Source: CAD feature listing. Evaluate the final solid. Frame: model axes, mm. A direction names the side the tool comes from. Coordinates: 2 decimals unless noted, no trailing zeros. Order: outer loops, then holes, each group sorted by start corner. A loop starts at its lowest first (then second) coordinate and runs counter-clockwise, first axis right, second up.
Autodesk Inventor part; units mm, degrees
ref_plane "YZ Plane" through (0, 0, 0) normal (1, 0, 0) x (0, 1, 0)
ref_plane "XZ Plane" through (0, 0, 0) normal (0, 1, 0) x (-1, 0, 0)
ref_plane "XY Plane" through (0, 0, 0) normal (0, 0, 1) x (1, 0, 0)
sketch "Sketch1" plane through (0, 0, 0) normal (0, 1, 0) x (-1, 0, 0)
  line L0 (0, 0) -> (0, -228.6)
  line L1 (0, -228.6) -> (-25.4, -228.6)
  line L2 (-25.4, -228.6) -> (-25.4, 10.5159)
  line L3 (-25.4, 10.5159) -> (24.2621, 60.178)
  line L4 (24.2621, 60.178) -> (42.5226, 42.5226)
  line L5 (42.5226, 42.5226) -> (0, 0)
  dimension "d0" = 228.6
  dimension "d1" = 25.4
  dimension "d2" = 135
  dimension "d3" = 25.4
extrude "Extrusion1" add sketch "Sketch1" along normal blind 25.4
sketch "Sketch2" plane through (0, 25.4, 0) normal (0, 1, 0) x (1, 0, 0)
  line L0 (25.4, 228.6) -> (0, 228.6)
  line L1 (9.525, 228.6) -> (0, 182.5245)
  line L2 (0, 228.6) -> (0, 0)
  dimension "d6" = 11.68
  dimension "d7" = 9.525
extrude "Extrusion2" cut sketch "Sketch2" against normal through all
shell "Shell1" thickness 3.175 removed faces 3 at (3.175, 16.9333, -197.883) at (14.8167, 8.4667, -228.6) at (-30.3489, 8.4667, 54.2929)
sketch "Sketch3" plane through (0, 25.4, 0) normal (0, 1, 0) x (1, 0, 0)
  circle A0 centre (-24.4095, -42.3701) radius 3.175
  line L0 (-42.5226, -42.5226) -> (-24.2621, -60.178)
  line L1 (0, 0) -> (-42.5226, -42.5226)
  line L2 (0, 0) -> (25.4, 0)
  line L3 (25.4, -10.5159) -> (25.4, 228.6)
  circle A1 centre (12.7, 12.7) radius 2.54
  line L4 (0, 182.5245) -> (0, 0)
  dimension "d11" = 6.35
  dimension "d12" = 12.7
  dimension "d13" = 12.7
  dimension "d14" = 5.08
  dimension "d15" = 12.7
  dimension "d16" = 12.7
extrude "Extrusion3" cut sketch "Sketch3" against normal through all
properties material "Aluminum 6061"
1. Section query C-C on x = 12.7. Return loops of the section in (y, z) (3 decimals).
Findings:
outline: (0, -228.6) - (3.175, -228.6) - (3.175, -15.24) - (0, -15.24) - close; (0, -10.16) - (3.175, -10.16) - (3.175, 18.726) - (22.225, 18.726) - (22.225, -10.16) - (25.4, -10.16) - (25.4, 23.216) - (0, 23.216) - close; (22.225, -228.6) - (25.4, -228.6) - (25.4, -15.24) - (22.225, -15.24) - close
2. Section query B-B on y = 8. Return loops of the section in (x, z) (1 decimal).
Findings:
outline: (-42.5, 42.5) - (0, 0) - (0, -182.5) - (3.2, -197.9) - (3.2, 1.3) - (-40.2, 44.7) - close; (-26.5, 58) - (22.2, 9.2) - (22.2, -228.6) - (25.4, -228.6) - (25.4, 10.5) - (-24.3, 60.2) - close
3. Access query for faces 1 (the face through (12.37, 23.83, -15.22)), 2 (the face through (22.225, 13, -111)), 3 (the face through (0, 13, -90)), 4 (the face through (7, 3.175, -85)). Directions: +Z, -Z, +X, -X, +Y, -Y. A direction counts if a zero-diameter tool reaches every point of the face in a straight line with its end or side. Return the directions, or none.
Findings:
face 1: +Y, -Y
face 2: -Z
face 3: -Z, -X, +Y, -Y
face 4: none
4. Pin query (flat end, axial travel): P1, Ø2, axis at y = 19.5, z = -152, coming from the -X side; P2, Ø6, axis at y = 21, z = 18.5, coming from the -X side; P3, Ø10, axis at x = 13, y = 4, coming from the +Z side. Return the tip coordinate at first contact, or that it passes through.
Findings:
P1: stops at x = 0
P2: stops at x = -21.5
P3: stops at z = 27.92
5. Section query D-D on x = -31. Return loops of the section in (y, z) (3 decimals), plus the area to 3 significant figures.
Findings:
outline: (0, 31) - (25.4, 31) - (25.4, 53.663) - (22.225, 53.663) - (22.225, 35.49) - (3.175, 35.49) - (3.175, 53.663) - (0, 53.663) - close
area: 229 mm2
6. Ray query, line 1 (X direction, y = 1.75, z = -12.7); line 2 (Y direction, x = 16, z = -155) (3 decimals). Return the intervals inside material, ascending.
Findings:
line 1: x = 0 to 10.16, 15.24 to 25.4
line 2: y = 0 to 3.175, 22.225 to 25.4
7. Section query A-A on z = -12.7. Return loops of the section in (x, y) (3 decimals), plus the area to 3 significant figures.
Findings:
outline: (0, 0) - (10.16, 0) - (10.16, 3.175) - (3.175, 3.175) - (3.175, 22.225) - (10.16, 22.225) - (10.16, 25.4) - (0, 25.4) - close; (15.24, 0) - (25.4, 0) - (25.4, 25.4) - (15.24, 25.4) - (15.24, 22.225) - (22.225, 22.225) - (22.225, 3.175) - (15.24, 3.175) - close
area: 250 mm2
8. Draft query along Z for faces 5 (the face through (12, 25.4, -84)), 6 (the face through (0.917, 12.522, 34.999)), 7 (the face through (-1.819, 12.567, 33.244)), 8 (the face through (-22, 13, 22)). Return one class per face: released by +Z, released by -Z, zero draft, split by the parting line, or undercut.
Findings:
face 5: zero draft
face 6: released by +Z
face 7: undercut
face 8: released by -Z
